Source: three-view drawing plus pictorial views. Frame: mm from the lowest corner of the part. A direction names the side the tool comes from. Give positions to 0.01 mm unless a question says otherwise; leave off trailing zeros. Loops run counter-clockwise (first coordinate to the right, second up) from the corner with the lowest first, then second, coordinate; pieces in that order, holes last. Notation, with made-up numbers: (78, 69.5) -> (82, 69.5) arc R25 cw to (82, 88.5) -> close; hole circle Ø8 at (-0.75, -37.75). An arc over 180 degrees is marked (long way). Answer as a JSON object with one key per item and string values. Group by question number.
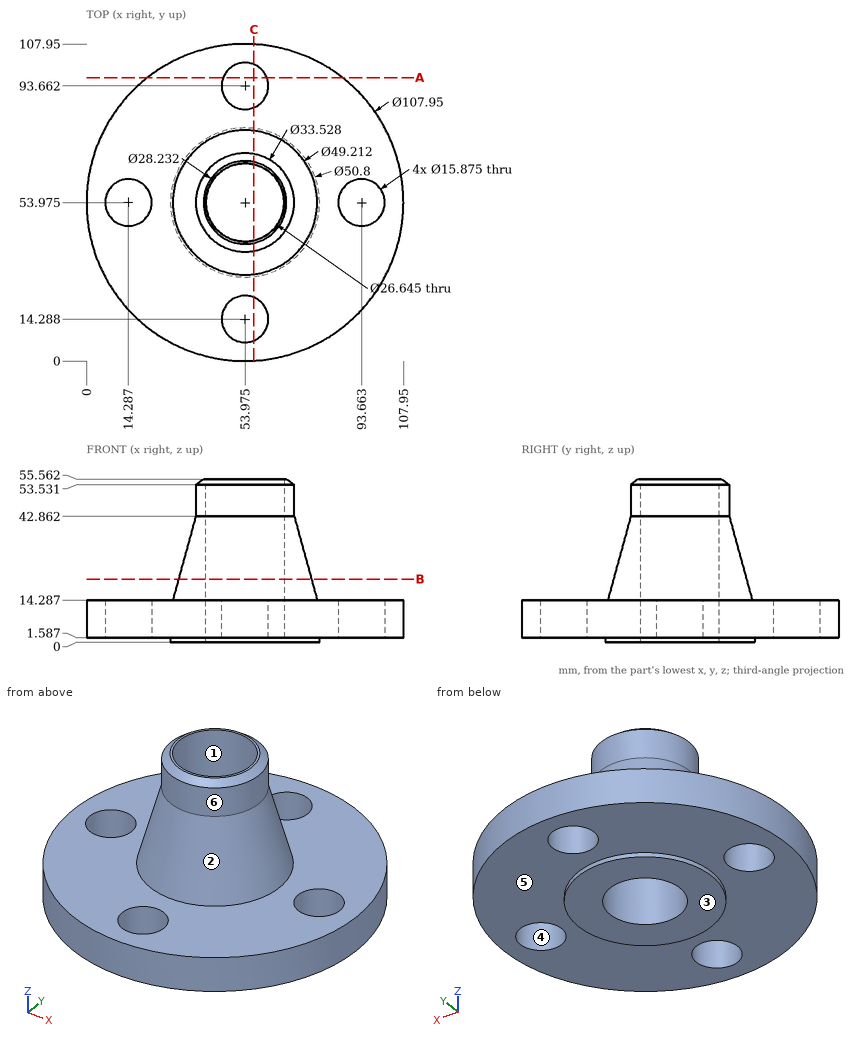
Q1. Section A-A on y = 96.5. Return the cut outline in (x, z) (1 decimal).
Q2. Section C-C on x = 57. State how many separate pieces and enclosed holes the cut face has, then the cut area to 3 significant figures.
Q3. Pull-direction query (Y, two-part tool) for the marked faces 1, 2 and 3; classes: +Y half, -Y half, draft (parallel to the pull), parting line (faces both ways), or undercut.
Q4. Ray query, probe 1 along Z at (x, y) = (58.5, 84); probe 2 along Y at (x, z) = (48, 36); probe 3 along X at (y, z) = (95, 10.5). Return the intervals inside material, ascending.
Q5. Section B-B on z = 21.5. Return the cut outline in (x, y) (1 decimal).
Q6. Pin query (flat end, axial travel): pin 1 Ø3 at (x, y) = (47, 41.5) entering from +Z; pin 2 Ø10 at (x, z) = (73.5, 16) entering from -Y; pin 3 Ø1 at (x, z) = (36.5, 21.5) entering from +Y; pin 4 Ø2 at (x, z) = (54.5, 36.5) entering from +Y. Return the tip coordinate at first contact, or that it passes through.
Q7. Set-up query: the marked faces 4, 5 and 6. Return all of +Z, -Z, +X, -X, +Y, -Y with unobstructed straight access to the full face (end or side cutting, diameter ignored); none if empty.
Numbers:
{
 "1": {"outline": "(20.7, 1.6) -> (46.6, 1.6) -> (46.6, 14.3) -> (20.7, 14.3) -> close; (61.4, 1.6) -> (87.2, 1.6) -> (87.2, 14.3) -> (61.4, 14.3) -> close"},
 "2": {"separate pieces": "4", "enclosed holes": "0", "area": "1,220 mm²"},
 "3": {"face 1": "undercut", "face 2": "parting line", "face 3": "draft"},
 "4": {"probe 1": "z = 1.59 to 14.29", "probe 2": "y = 36.31 to 42.07, 65.88 to 71.64", "probe 3": "x = 18.9 to 46.15, 61.8 to 89.05"},
 "5": {"outline": "circle Ø45.3 at (54, 54); hole circle Ø26.6 at (54, 54)"},
 "6": {"pin 1": "stops at z = 55.56", "pin 2": "stops at y = 2.08", "pin 3": "stops at y = 68.97", "pin 4": "stops at y = 72.75"},
 "7": {"face 4": "+Z, -Z", "face 5": "-Z", "face 6": "+Z"}
}
